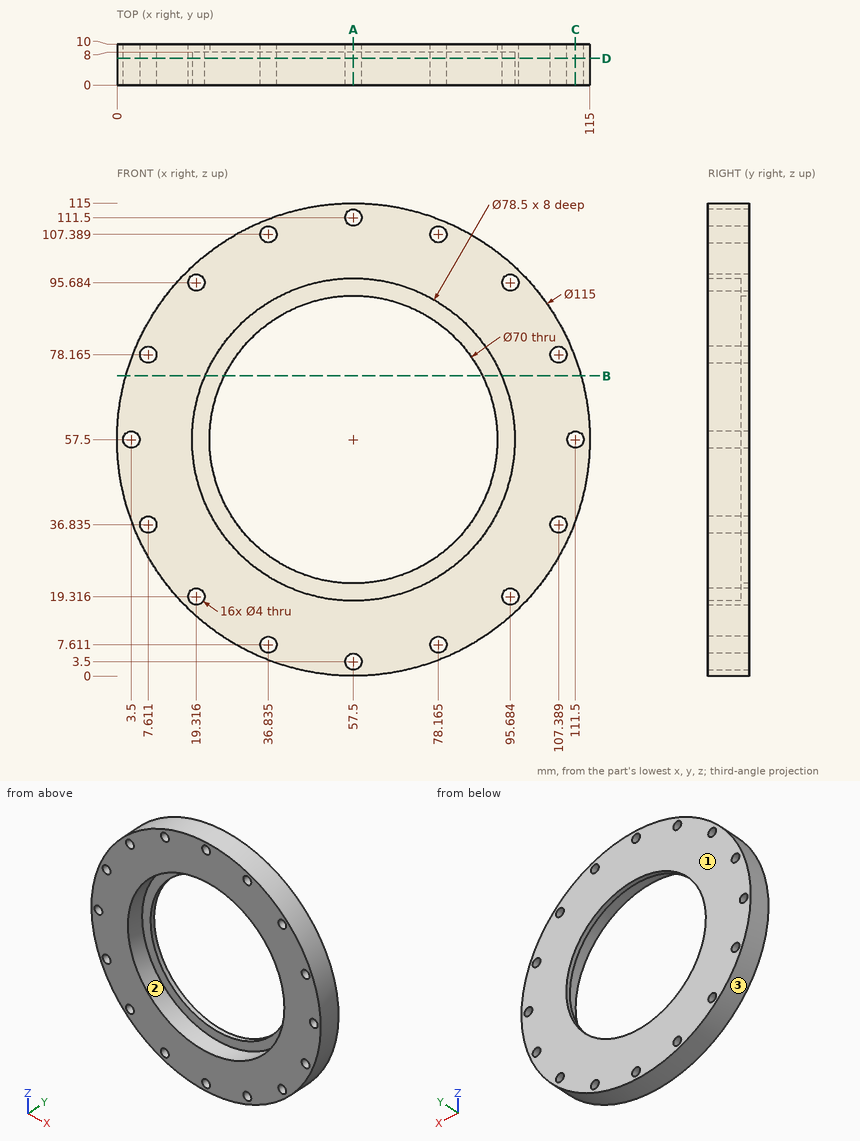
Drawing for the job (mm, zero at the part's lowest x, y, z). Give positions to 0.01 mm unless a question says otherwise; leave off trailing zeros. Loops run counter-clockwise (first coordinate to the right, second up) from the corner with the lowest first, then second, coordinate; pieces in that order, holes last.
1) Two-plate mould, pull along Z, no slides. Class the marked faces 1, 2 and 3: released by +Z, released by -Z, zero draft, split by the parting line, or undercut.
Values follow:
face 1: zero draft
face 2: undercut
face 3: split by the parting line
2) Drop flat-ended pins along their axis: P1, Ø3, axis at x = 111.5, z = 57.5, coming from the -Y side; P2, Ø2, axis at x = 74, y = 8, coming from the +Z side; P3, Ø1, axis at y = 3, z = 39.5, coming from the +X side; P4, Ø1, axis at y = 8, z = 55.5, coming from the -X side. Give the stop position or say it passes through.
Values follow:
P1: passes through
P2: stops at z = 112.87
P3: stops at x = 112.27
P4: stops at x = 0.02
3) Probe line 1 along X through (y, z) = (4.5, 57.5); line 2 along X through (y, z) = (7, 35.5) (1 decimal); line 3 along Z through (x, y) = (21, 1.75) (1 decimal). List the from-to ranges inside material, lowest first.
Values follow:
line 1: x = 0 to 1.5, 5.5 to 18.25, 96.75 to 109.5, 113.5 to 115
line 2: x = 4.4 to 6.1, 9.1 to 25, 90 to 105.9, 108.9 to 110.6
line 3: z = 13.1 to 18.2, 20.4 to 43.1, 71.9 to 94.6, 96.8 to 101.9
4) Band-saw the part on D-D on y = 6.5. State how many separate pieces and enclosed holes the cut face has, then the cut area to 3 significant figures.
Values follow:
separate pieces: 1
enclosed holes: 17
area: 5,350 mm2
5) Band-saw the part on C-C on x = 111.5. List the corners of the cut face in (y, z) (1 decimal).
Values follow:
outline: (0, 37.7) - (10, 37.7) - (10, 55.5) - (0, 55.5) - close; (0, 59.5) - (10, 59.5) - (10, 77.3) - (0, 77.3) - close
6) Band-saw the part on A-A on x = 57.5. List the corners of the cut face in (y, z).
Values follow:
outline: (0, 0) - (10, 0) - (10, 1.5) - (0, 1.5) - close; (0, 5.5) - (10, 5.5) - (10, 22.5) - (8, 22.5) - (8, 18.25) - (0, 18.25) - close; (0, 96.75) - (8, 96.75) - (8, 92.5) - (10, 92.5) - (10, 109.5) - (0, 109.5) - close; (0, 113.5) - (10, 113.5) - (10, 115) - (0, 115) - close
7) Band-saw the part on B-B on z = 73. List the corners of the cut face in (x, y).
Values follow:
outline: (2.13, 0) - (21.44, 0) - (21.44, 8) - (26.12, 8) - (26.12, 10) - (2.13, 10) - close; (88.88, 8) - (93.56, 8) - (93.56, 0) - (112.87, 0) - (112.87, 10) - (88.88, 10) - close
